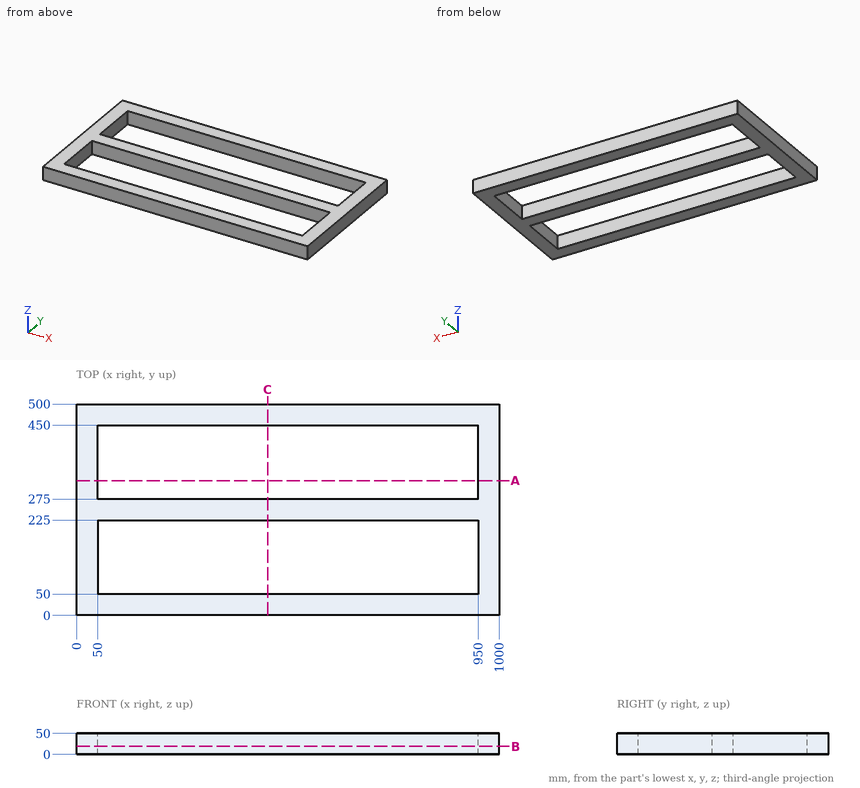
Design review of the part shown in the three views and the two pictorial views. Dimensions are in mm from the part's minimum x, y and z. Give positions to 0.01 mm unless a question says otherwise; leave off trailing zeros. Loops run counter-clockwise (first coordinate to the right, second up) from the corner with the lowest first, then second, coordinate; pieces in that order, holes last. Notation, with made-up numbers: M 25,-34 L 66,-34 A30 ccw 66,0 Z; hole C -24.5,11.25 d9. An arc over 180 degrees is marked long. Put each result on its own line as item: value. Start each with the question number.
(1) Add section A-A, the plane y = 319. Write out the cut boundary in (x, z), then the cut area to 3 significant figures.
(2) Add section B-B, the plane z = 19. Write out the cut boundary in (x, y), then the cut area to 3 significant figures.
(3) Wall thickness on L1, parallel to Y at x = 714, z = 38; L2, parallel to X at y = 419, z = 40.5: over which ranges is each line inside the solid? List them lowest first.
(4) Add section C-C, the plane x = 452. Write out the cut boundary in (y, z).
Result:
1. outline: M 0,0 L 50,0 L 50,50 L 0,50 Z; M 950,0 L 1000,0 L 1000,50 L 950,50 Z
1. area: 5,000 mm^2
2. outline: M 0,0 L 1000,0 L 1000,500 L 0,500 Z; hole M 50,50 L 950,50 L 950,225 L 50,225 Z; hole M 50,275 L 950,275 L 950,450 L 50,450 Z
2. area: 185,000 mm^2
3. L1: y = 0 to 50, 225 to 275, 450 to 500
3. L2: x = 0 to 50, 950 to 1000
4. outline: M 0,0 L 50,0 L 50,50 L 0,50 Z; M 225,0 L 275,0 L 275,50 L 225,50 Z; M 450,0 L 500,0 L 500,50 L 450,50 Z
